```python
from build123d import *

# Parameters (mm, degrees)
IZIM1_R             = 1.55
IZIM1_W             = 120
IZIM1_H             = 10
BOSS_EXTRUDE2_DEPTH = 10


with BuildPart() as part:
    # Çizim1 → Boss-Extrude2 (new body)
    with BuildSketch(Plane.XY):
        Polygon((-130, -250), (-130, -240), (-10, -240), (-10, -250), (10, -250), (10, -240), (130, -240), (130, -250), (190, -250), (190, 0), (-190, 0), (-190, -250), align=None)
        with Locations((-141.295330694, -245)):
            Circle(IZIM1_R, mode=Mode.SUBTRACT)
        with Locations((-141.295330694, -205)):
            Circle(IZIM1_R, mode=Mode.SUBTRACT)
        with Locations((-70, -205)):
            Rectangle(IZIM1_W, IZIM1_H, mode=Mode.SUBTRACT)
        with Locations((-1.295330694, -245)):
            Circle(IZIM1_R, mode=Mode.SUBTRACT)
        with Locations((-1.295330694, -205)):
            Circle(IZIM1_R, mode=Mode.SUBTRACT)
        with Locations((70, -205)):
            Rectangle(IZIM1_W, IZIM1_H, mode=Mode.SUBTRACT)
        with Locations((138.704669306, -245)):
            Circle(IZIM1_R, mode=Mode.SUBTRACT)
        with Locations((138.704669306, -205)):
            Circle(IZIM1_R, mode=Mode.SUBTRACT)
    extrude(amount=BOSS_EXTRUDE2_DEPTH)


solid = part.part
```
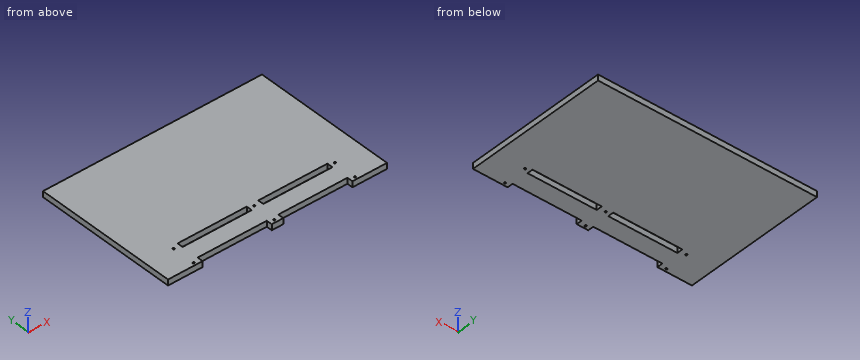
Could you check a few things on this model? Use its own coordinates, in mm. Give positions to 0.01 mm unless a question says otherwise; leave off trailing zeros. Write each loop counter-clockwise with the first axis right and the second up, starting at its lowest first coordinate (ties: lowest second). Pieces come first, ordered by that corner, then holes. Notation, with made-up numbers: (28.25, 0.25) - (59.25, 0.25) arc R24 ccw to (59.25, 21.25) - close; hole circle Ø8 at (0, 43). An arc over 180 degrees is marked (long way). One line per item, written item: value. Start each with the question number.
Item 1: I'm going to push a flat-ended pin straight in: pin 1 (5 mm diameter, centred on x = -1.3, y = -205, fed in from +Z). Where does the tip first touch, or does it pass through?
Item 2: Imagine slicing it at B-B, the plane z = 5.5. Give the number of separate pieces and of enclosed holes in the cut face, and give its area (3 significant figures).
Item 3: Please list where these lines run through material, in increasing order: line 1 (X direction, y = -245, z = 8); line 2 (Y direction, x = 26, z = 7). Write a range as from..to.
Item 4: Imagine slicing it at A-A, the plane x = 81.5. List the corners of the cut face in (y, z) for me, and give its area (3 significant figures).
Geometry says:
1. pin 1: z = 10
2. separate pieces: 1
2. enclosed holes: 8
2. area: 90,200 mm^2
3. line 1: -190..-142.85, -139.75..-130, -10..-2.85, 0.25..10, 130..137.15, 140.25..190
3. line 2: -240..-210, -200..0
4. outline: (-240, 0) - (-210, 0) - (-210, 10) - (-240, 10) - close; (-200, 0) - (0, 0) - (0, 10) - (-200, 10) - close
4. area: 2,300 mm^2
